Autodesk Inventor part; units mm, degrees
ref_plane "YZ Plane" through (0, 0, 0) normal (1, 0, 0) x (0, 1, 0)
ref_plane "XZ Plane" through (0, 0, 0) normal (0, 1, 0) x (-1, 0, 0)
ref_plane "XY Plane" through (0, 0, 0) normal (0, 0, 1) x (1, 0, 0)
sketch "スケッチ1" plane through (0, 0, 0) normal (1, 0, 0) x (0, 1, 0)
  circle A0 centre (0, 0) radius 4
  circle A1 centre (30, -300) radius 4
  circle A2 centre (230, 350) radius 4
  line L0 (248.6746, 396.6269) -> (151.2885, -136.9946)
  line L1 (151.2885, -136.9946) -> (22.8179, -328.6776)
  line L2 (22.8179, -328.6776) -> (-10.3029, 2.5306)
  line L3 (248.6746, 396.6269) -> (-10.3029, 2.5306)
  dimension "d0" = 30
  dimension "d1" = 300
  dimension "d2" = 8
  dimension "d3" = 8
  dimension "d4" = 350
  dimension "d5" = 230
  dimension "d6" = 8
  dimension "d9" = 10
  dimension "d11" = 10
  dimension "d13" = 10
  dimension "d14" = 10
  dimension "d16" = 10
  dimension "d29" = 10
extrude "押し出し3" add sketch "スケッチ1" along normal mid plane 5
fillet "フィレット3" radius 10 3 edges at (0, 248.6746, 396.6269) (0, 22.8179, -328.6776) (0, -10.3029, 2.5306)
properties part number "swan_plate"
CAD build for the part. Positions are in the model's coordinates, mm. Round coordinates to 2 decimals unless told otherwise and drop trailing zeros. Order: outer loops, then holes, each group sorted by start corner. A loop starts at its lowest first (then second) coordinate and runs counter-clockwise, first axis right, second up.
Item 1: Pin check, flat tips, straight feed: pin 1 (3 mm diameter, centred on x = -1, y = 37.5, fed in from -Z); pin 2 (2 mm diameter, centred on x = 1.5, y = 129.5, fed in from +Z); pin 3 (3 mm diameter, centred on x = -2, z = -209, fed in from +Y). Stop position of each tip, or through.
Item 2: Saw through at A-A on x = -0.4. Write the cut outline in (y, z).
Item 3: Saw through at B-B on z = 301. Write the cut outline in (x, y).
Item 4: Saw through at C-C on y = 96.5. Write the cut outline in (x, z).
Item 5: Probe line 1 along Y through (x, z) = (0.7, -300); line 2 along Z through (x, y) = (-0.95, 30); line 3 along Y through (x, z) = (0.55, 350). List the from-to ranges inside material, lowest first.
Reported:
1. pin 1: stops at z = -308
1. pin 2: stops at z = 216.8
1. pin 3: stops at y = 104.03
2. outline: (-9.95, -1) - (20.05, -301) arc R10 ccw to (38.31, -305.57) - (151.29, -136.99) - (239.84, 348.2) arc R10 ccw to (221.64, 355.49) - (-8.36, 5.49) arc R10 ccw to start; hole circle Ø8 at (0, 0); hole circle Ø8 at (30, -300); hole circle Ø8 at (230, 350)
3. outline: (-2.5, 185.83) - (2.5, 185.83) - (2.5, 231.22) - (-2.5, 231.22) - close
4. outline: (-2.5, -218.74) - (2.5, -218.74) - (2.5, 165.06) - (-2.5, 165.06) - close
5. line 1: y = 19.95 to 26, 34 to 42.04
5. line 2: z = -310 to -304, -296 to 63.86
5. line 3: y = 218.03 to 226, 234 to 240
